from build123d import *

# Parameters (mm, degrees)
F0_R      = 1.75
F0_R_2    = 3.25
F1_DEPTH  = 4
F2_R      = 2
F3_DEPTH  = 34
F5_R      = 6
F6_DEPTH  = 40
F7_R      = 4
F8_DEPTH  = 40
F10_R     = 6
F10_R_2   = 2.6
F11_DEPTH = 2
F12_W     = 8.5
F12_H     = 2
F13_DEPTH = 10


with BuildPart() as f1:
    # F0 (on Top) → F1 (new body)
    with BuildSketch(Plane.XY):
        with BuildLine():
            ThreePointArc((-17, -13), (-15.828427, -15.828427), (-13, -17))
            Line((-13, -17), (13, -17))
            ThreePointArc((13, -17), (15.828427, -15.828427), (17, -13))
            Line((17, -13), (17, 13))
            ThreePointArc((17, 13), (15.828427, 15.828427), (13, 17))
            Line((13, 17), (-13, 17))
            ThreePointArc((-13, 17), (-15.828427, 15.828427), (-17, 13))
            Line((-17, 13), (-17, -13))
        make_face()
        with Locations((-13, -13)):
            Circle(F0_R, mode=Mode.SUBTRACT)
        with Locations((-7, -7)):
            Circle(F0_R_2, mode=Mode.SUBTRACT)
        with Locations((13, -13)):
            Circle(F0_R, mode=Mode.SUBTRACT)
        with Locations((7, -7)):
            Circle(F0_R_2, mode=Mode.SUBTRACT)
        with Locations((-7, 7)):
            Circle(F0_R_2, mode=Mode.SUBTRACT)
        with Locations((-13, 13)):
            Circle(F0_R, mode=Mode.SUBTRACT)
        with Locations((7, 7)):
            Circle(F0_R_2, mode=Mode.SUBTRACT)
        with Locations((13, 13)):
            Circle(F0_R, mode=Mode.SUBTRACT)
    extrude(amount=F1_DEPTH)


with BuildPart() as f3:
    # F2 (on face) → F3 (new body)
    with BuildSketch(Plane.XZ.offset(17)):
        Circle(F2_R)
    extrude(amount=-F3_DEPTH)


with BuildPart() as f1_1:
    add(f1.part)

    # F4: cut F3
    add(f3.part, mode=Mode.SUBTRACT)

    # F5 (on face) → F6 (join)
    with BuildSketch(Plane.XY.offset(4)):
        Circle(F5_R)
    extrude(amount=F6_DEPTH)


with BuildPart() as f8:
    # F7 (on face) → F8 (new body)
    with BuildSketch(Plane.XY.offset(44)):
        Circle(F7_R)
    extrude(amount=-F8_DEPTH)


with BuildPart() as f1_2:
    add(f1_1.part)

    # F9: cut F8
    add(f8.part, mode=Mode.SUBTRACT)

    # F10 (on face) → F11 (join)
    with BuildSketch(Plane.XY.offset(44)):
        Circle(F10_R)
        Circle(F10_R_2, mode=Mode.SUBTRACT)
    extrude(amount=F11_DEPTH)


with BuildPart() as f13:
    # F12 (on face) → F13 (new body)
    with BuildSketch(Plane.XY.offset(4)):
        Rectangle(F12_W, F12_H)
    extrude(amount=-F13_DEPTH)


with BuildPart() as f1_3:
    add(f1_2.part)

    # F14: cut F13
    add(f13.part, mode=Mode.SUBTRACT)


solid = f1_3.part
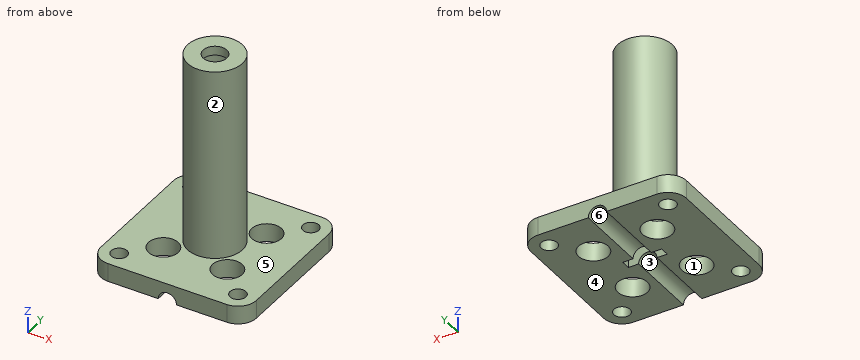
Part model, mm, in its own coordinate system. Face numbers are marked on the shaded views. A direction names the side the tool comes from. Give positions to 0.01 mm unless a question says otherwise; leave off trailing zeros. Loops run counter-clockwise (first coordinate to the right, second up) from the corner with the lowest first, then second, coordinate; pieces in that order, holes last. Notation, with made-up numbers: M 18.25,49 L 22.25,49 A19 cw 22.25,62 Z; hole C 73.5,9.5 d3. An arc over 180 degrees is marked long. Put each result on its own line as item: value. Start each with the question number.
1) Probe probe 1 along Y at (x, z) = (-7, 2.15); probe 2 along Y at (x, z) = (-13, 3.15); probe 3 along Y at (x, z) = (4, 3). List the from-to ranges inside material, lowest first.
2) Flat gauge pins, fed straight in: pin 1 (8 mm diameter, centred on x = -6.5, z = 15.5, fed in from -Y); pin 2 (5.5 mm diameter, centred on x = -13, y = -13, fed in from +Z); pin 3 (3 mm diameter, centred on y = 6.5, z = 16.5, fed in from +X). Where does each tip first touch, or does it go through?
3) Saw through at D-D (x = -7). List the corners of the cut face in (y, z).
4) 3-axis set-ups, long thin cutter, end or side, ignore diameter. For the marked faces 5 and 6: which of +Z, -Z, +X, -X, +Y, -Y reach the whole face in a straight line?
5) Saw through at C-C (y = -7). List the corners of the cut face in (x, z).
6) Saw through at B-B (y = 0). List the corners of the cut face in (x, z).
7) Pull direction X, two halves, no side cores. Call the marked faces 1, 2, 3 and 4: +X half, -X half, draft (parallel to the pull), parting line (faces both ways), or undercut.
8) Saw through at A-A (x = 0). List the corners of the cut face in (y, z), then the cut area to 3 significant figures.
Numbers:
1. probe 1: -17 to -10.25, -3.75 to 3.75, 10.25 to 17
1. probe 2: -17 to -14.75, -11.25 to 11.25, 14.75 to 17
1. probe 3: -17 to -8.25, -5.75 to -1, 1 to 5.75, 8.25 to 17
2. pin 1: y = -5.45
2. pin 2: z = 4
2. pin 3: x = 3.32
3. outline: M -17,0 L -10.25,0 L -10.25,4 L -17,4 Z; M -3.75,0 L 3.75,0 L 3.75,4 L -3.75,4 Z; M 10.25,0 L 17,0 L 17,4 L 10.25,4 Z
4. face 5: +Z
4. face 6: -Z, +Y, -Y
5. outline: M -17,0 L -10.25,0 L -10.25,4 L -17,4 Z; M -3.75,0 L -2,0 A2 cw 2,0 L 3.75,0 L 3.75,4 L -3.75,4 Z; M 10.25,0 L 17,0 L 17,4 L 10.25,4 Z
6. outline: M -17,0 L -4.25,0 L -4.25,4 L -4,4 L -4,44 L -2.6,44 L -2.6,46 L -6,46 L -6,4 L -17,4 Z; M 2.6,44 L 4,44 L 4,4 L 4.25,4 L 4.25,0 L 17,0 L 17,4 L 6,4 L 6,46 L 2.6,46 Z
7. face 1: undercut
7. face 2: parting line
7. face 3: undercut
7. face 4: draft
8. outline: M -17,2 L -1,2 L -1,4 L -4,4 L -4,44 L -2.6,44 L -2.6,46 L -6,46 L -6,4 L -17,4 Z; M 1,2 L 17,2 L 17,4 L 6,4 L 6,46 L 2.6,46 L 2.6,44 L 4,44 L 4,4 L 1,4 Z
8. area: 238 mm^2
